Build history of the part. All positions in model axes, mm. Round coordinates to 2 decimals unless told otherwise and drop trailing zeros. Order: outer loops, then holes, each group sorted by start corner. A loop starts at its lowest first (then second) coordinate and runs counter-clockwise, first axis right, second up. Notation, with made-up numbers: (46, -29) -> (59, -29) arc R13 cw to (59, -21) -> close; hole circle Ø1 at (45, 1). An arc over 180 degrees is marked (long way). Use a Markdown table: item, result. Add a question column.
Item 1: Slice it at A-A, the plane x = 0. Give the cut face in (y, z), plus the area to 3 significant figures.
Item 2: Two-plate mould, pull along X, no slides. Class faces 1 (the face through (-1, 2, 0)), 2 (the face through (64.592, 0.601, 2.465)), 3 (the face through (71.297, 3.859, 2.535)): released by +X, released by -X, zero draft, split by the parting line, or undercut.
Item 3: Slice it at B-B, the plane z = 1.4. Give the cut face in (x, y).
Item 4: Probe L1, parallel to X at y = -0.25, z = 2.85; L2, parallel to Y at x = -66.5, z = 2; L3, parallel to X at y = -0.5, z = 1.45. List the from-to ranges inside material, lowest first.
from build123d import *

# Parameters (mm, degrees)
SZKIC1_W                    = 145
SZKIC1_H                    = 10
DODANIE_WYCI_GNI_CIE1_DEPTH = 5
OTWORY_USTALAJ_CE_4_0MM1_D  = 4
ZAOKR_GLENIE1_R             = 4


with BuildPart() as part:
    # Szkic1 → Dodanie-wyciągnięcie1 (new body)
    with BuildSketch(Plane.XY):
        Rectangle(SZKIC1_W, SZKIC1_H)
    extrude(amount=DODANIE_WYCI_GNI_CIE1_DEPTH)

    # Otwory ustalające Ø4.0mm1 (through all)
    with Locations(Plane.XY.offset(5)):
        with Locations((0, 0), (-66.5, 0), (66.5, 0)):
            Hole(OTWORY_USTALAJ_CE_4_0MM1_D / 2)

    # Zaokrąglenie1
    zaokr_glenie1_edges = [part.edges().sort_by_distance(p)[0] for p in [
        (72.5, -5, 2.5),
        (-72.5, -5, 2.5),
        (-72.5, 5, 2.5),
        (72.5, 5, 2.5),
    ]]
    fillet(zaokr_glenie1_edges, radius=ZAOKR_GLENIE1_R)


solid = part.part
Check sheet entries:
| question | item | result |
|---|---|---|
| 1 | outline | (-5, 0) -> (-2, 0) -> (-2, 5) -> (-5, 5) -> close; (2, 0) -> (5, 0) -> (5, 5) -> (2, 5) -> close |
| 1 | area | 30.0 mm2 |
| 2 | face 1 | zero draft |
| 2 | face 2 | undercut |
| 2 | face 3 | released by +X |
| 3 | outline | (-72.5, -1) arc R4 ccw to (-68.5, -5) -> (68.5, -5) arc R4 ccw to (72.5, -1) -> (72.5, 1) arc R4 ccw to (68.5, 5) -> (-68.5, 5) arc R4 ccw to (-72.5, 1) -> close; hole circle Ø4 at (-66.5, 0); hole circle Ø4 at (0, 0); hole circle Ø4 at (66.5, 0) |
| 4 | L1 | -72.5 to -68.48, -64.52 to -1.98, 1.98 to 64.52, 68.48 to 72.5 |
| 4 | L2 | -5 to -2, 2 to 5 |
| 4 | L3 | -72.5 to -68.44, -64.56 to -1.94, 1.94 to 64.56, 68.44 to 72.5 |
